Read the model definition and answer for the solid it produces. Units are mm, in the model's axes. Coordinates: 2 decimals unless noted, no trailing zeros. Write each loop counter-clockwise with the first axis right and the second up, starting at its lowest first coordinate (ties: lowest second). Pieces come first, ordered by that corner, then holes. Notation, with made-up numbers: (52, 19.5) -> (82, 19.5) arc R24 cw to (82, 54.5) -> close; hole circle Ø3 at (14, 65.5). An arc over 180 degrees is marked (long way). Return JSON: item names as keys, results as strings.
from build123d import *

# Parameters (mm, degrees)
F0_R      = 1.25
F1_DEPTH  = 6
F2_DEPTH  = 50
F3_DEPTH  = 50
F4_R      = 1.25
F5_DEPTH  = 6
F6_R      = 1.25
F7_DEPTH  = 6
F9_DEPTH  = 2
F11_DEPTH = 1.5
F10_W     = 6
F10_H     = 6
F12_DEPTH = 6
F13_R     = 1.25
F14_DEPTH = 30


with BuildPart() as f1:
    # F0 (on Top) → F1 (new body)
    with BuildSketch(Plane.XY):
        with BuildLine():
            ThreePointArc((10, -3), (12.1213203436, -2.1213203436), (13, 0))
            ThreePointArc((13, 0), (12.1213203436, 2.1213203436), (10, 3))
            ThreePointArc((10, 3), (7.8786796564, 2.1213203436), (7, 0))
            ThreePointArc((7, 0), (7.8786796564, -2.1213203436), (10, -3))
        make_face()
        with Locations((10, 0)):
            Circle(F0_R, mode=Mode.SUBTRACT)
        with BuildLine():
            ThreePointArc((7, 0), (7.8786796564, 2.1213203436), (10, 3))
            Line((10, 3), (7, 3))
            Line((7, 3), (7, 0))
        make_face()
        with BuildLine():
            Line((7, -3), (10, -3))
            ThreePointArc((10, -3), (7.8786796564, -2.1213203436), (7, 0))
            Line((7, 0), (7, -3))
        make_face()
        with BuildLine():
            Line((13, -3), (13, 0))
            ThreePointArc((13, 0), (12.1213203436, -2.1213203436), (10, -3))
            Line((10, -3), (13, -3))
        make_face()
        with BuildLine():
            ThreePointArc((10, 3), (12.1213203436, 2.1213203436), (13, 0))
            Line((13, 0), (13, 3))
            Line((13, 3), (10, 3))
        make_face()
        with Locations((10, 0)):
            Circle(F0_R)
    extrude(amount=F1_DEPTH)

    # F0 (on Top) → F2 (join)
    with BuildSketch(Plane.XY):
        with BuildLine():
            ThreePointArc((10, -3), (12.1213203436, -2.1213203436), (13, 0))
            ThreePointArc((13, 0), (12.1213203436, 2.1213203436), (10, 3))
            ThreePointArc((10, 3), (7.8786796564, 2.1213203436), (7, 0))
            ThreePointArc((7, 0), (7.8786796564, -2.1213203436), (10, -3))
        make_face()
        with Locations((10, 0)):
            Circle(F0_R, mode=Mode.SUBTRACT)
    extrude(amount=F2_DEPTH)

    # F4 (on face) → F5 (cut)
    with BuildSketch(Plane.YZ.offset(13)):
        with Locations((0, 3)):
            Circle(F4_R)
        with BuildLine():
            Line((-3, 0), (0, 0))
            ThreePointArc((0, 0), (-2.1213203436, 0.8786796564), (-3, 3))
            Line((-3, 3), (-3, 0))
        make_face()
        with BuildLine():
            Line((3, 0), (3, 3))
            ThreePointArc((3, 3), (2.1213203436, 0.8786796564), (0, 0))
            Line((0, 0), (3, 0))
        make_face()
    extrude(amount=-F5_DEPTH, mode=Mode.SUBTRACT)



with BuildPart() as f1b:
    # F0 (on Top) → F1, piece 2 (new body)
    with BuildSketch(Plane.XY):
        with BuildLine():
            ThreePointArc((-10, 3), (-7.8786796564, 2.1213203436), (-7, 0))
            Line((-7, 0), (-7, 3))
            Line((-7, 3), (-10, 3))
        make_face()
        with BuildLine():
            ThreePointArc((-13, 0), (-12.1213203436, 2.1213203436), (-10, 3))
            Line((-10, 3), (-13, 3))
            Line((-13, 3), (-13, 0))
        make_face()
        with BuildLine():
            ThreePointArc((-10, -3), (-7.8786796564, -2.1213203436), (-7, 0))
            ThreePointArc((-7, 0), (-7.8786796564, 2.1213203436), (-10, 3))
            ThreePointArc((-10, 3), (-12.1213203436, 2.1213203436), (-13, 0))
            ThreePointArc((-13, 0), (-12.1213203436, -2.1213203436), (-10, -3))
        make_face()
        with Locations((-10, 0)):
            Circle(F0_R, mode=Mode.SUBTRACT)
        with BuildLine():
            Line((-13, -3), (-10, -3))
            ThreePointArc((-10, -3), (-12.1213203436, -2.1213203436), (-13, 0))
            Line((-13, 0), (-13, -3))
        make_face()
        with BuildLine():
            Line((-7, -3), (-7, 0))
            ThreePointArc((-7, 0), (-7.8786796564, -2.1213203436), (-10, -3))
            Line((-10, -3), (-7, -3))
        make_face()
        with Locations((-10, 0)):
            Circle(F0_R)
    extrude(amount=F1_DEPTH)

    # F0 (on Top) → F3 (join)
    with BuildSketch(Plane.XY):
        with BuildLine():
            ThreePointArc((-10, -3), (-7.8786796564, -2.1213203436), (-7, 0))
            ThreePointArc((-7, 0), (-7.8786796564, 2.1213203436), (-10, 3))
            ThreePointArc((-10, 3), (-12.1213203436, 2.1213203436), (-13, 0))
            ThreePointArc((-13, 0), (-12.1213203436, -2.1213203436), (-10, -3))
        make_face()
        with Locations((-10, 0)):
            Circle(F0_R, mode=Mode.SUBTRACT)
    extrude(amount=F3_DEPTH)

    # F6 (on face) → F7 (cut)
    with BuildSketch(Plane(origin=(-13, 0, 0), x_dir=(0, -1, 0), z_dir=(-1, 0, 0))):
        with Locations((0, 3)):
            Circle(F6_R)
        with BuildLine():
            Line((-3, 0), (0, 0))
            ThreePointArc((0, 0), (-2.1213203436, 0.8786796564), (-3, 3))
            Line((-3, 3), (-3, 0))
        make_face()
        with BuildLine():
            Line((3, 0), (3, 3))
            ThreePointArc((3, 3), (2.1213203436, 0.8786796564), (0, 0))
            Line((0, 0), (3, 0))
        make_face()
    extrude(amount=-F7_DEPTH, mode=Mode.SUBTRACT)


with BuildPart() as f9:
    # F8 (on Front) → F9 (new body, symmetric)
    with BuildSketch(Plane.XZ):
        Polygon((-10, 7), (10, 7), (10, 11), (7.5421927808, 11), (-7.5421927808, 11), (-10, 11), align=None)
    extrude(amount=F9_DEPTH, both=True)


with BuildPart() as f1_1:
    add(f1.part)

    add(f1b.part)  # F11 merges F1b

    add(f9.part)  # F11 merges F9
    # F8 (on Front) → F11 (join, symmetric)
    with BuildSketch(Plane.XZ):
        Polygon((-10, 39), (-10, 35.5590698932), (-2.4578072192, 25), (0, 28.4409301068), (-7.5421927808, 39), align=None)
        Polygon((-2.4578072192, 25), (0, 21.5590698932), (2.4578072192, 25), (0, 28.4409301068), align=None)
        Polygon((7.5421927808, 11), (10, 11), (10, 14.4409301068), (2.4578072192, 25), (0, 21.5590698932), align=None)
        Polygon((-10, 14.4409301068), (-10, 11), (-7.5421927808, 11), (0, 21.5590698932), (-2.4578072192, 25), align=None)
        Polygon((2.4578072192, 25), (10, 35.5590698932), (10, 39), (7.5421927808, 39), (0, 28.4409301068), align=None)
        Polygon((7.5421927808, 39), (10, 39), (10, 43), (-10, 43), (-10, 39), (-7.5421927808, 39), align=None)
    extrude(amount=F11_DEPTH, both=True)

    # F10 (on face) → F12 (join)
    with BuildSketch(Plane.XY.offset(50)):
        with Locations((-10, 0)):
            Rectangle(F10_W, F10_H)
        with Locations((10, 0)):
            Rectangle(F10_W, F10_H)
    extrude(amount=-F12_DEPTH)

    # F13 (on face) → F14 (cut)
    with BuildSketch(Plane.YZ.offset(13)):
        with Locations((0, 47)):
            Circle(F13_R)
        with BuildLine():
            Line((-3, 50), (-3, 47))
            ThreePointArc((-3, 47), (-2.1213203436, 49.1213203436), (0, 50))
            Line((0, 50), (-3, 50))
        make_face()
        with BuildLine():
            ThreePointArc((0, 50), (2.1213203436, 49.1213203436), (3, 47))
            Line((3, 47), (3, 50))
            Line((3, 50), (0, 50))
        make_face()
    extrude(amount=-F14_DEPTH, mode=Mode.SUBTRACT)


solid = f1_1.part
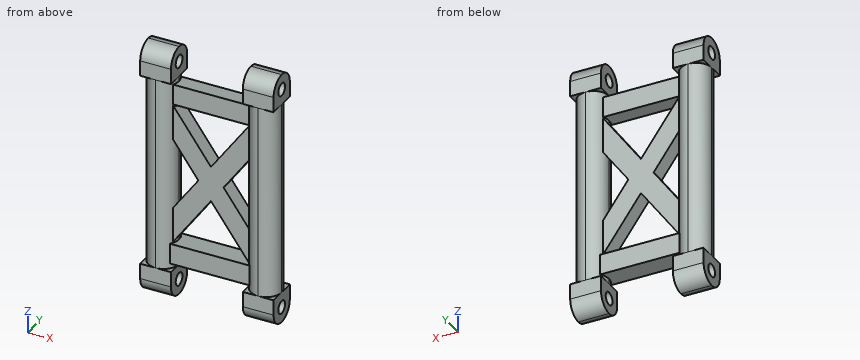
1. Consider L1, parallel to X at y = -0.25, z = 19; L2, parallel to Y at x = -10, z = 25.5; L3, parallel to X at y = -1, z = 19.5. Determine where each line is inside the solid, lowest interval first.
Taken from the geometry:
{"L1": "x = -12.99 to -11.22, -8.78 to -7.01, -6.74 to -1.83, 1.83 to 6.74, 7.01 to 8.78, 11.22 to 12.99", "L2": "y = -3 to -1.25, 1.25 to 3", "L3": "x = -12.83 to -10.75, -9.25 to -7.17, -6.39 to -1.47, 1.47 to 6.39, 7.17 to 9.25, 10.75 to 12.83"}
2. The part is cut by section D-D (z = 17.5). Determine the outline of the cut face in (x, y), then the cut area to 3 significant figures.
Taken from the geometry:
{"outline": "(-7.4, -1.5) -> (-2.9, -1.5) -> (-2.9, 1.5) -> (-7.4, 1.5) arc R3 ccw (long way) to start; (2.9, -1.5) -> (7.4, -1.5) arc R3 ccw (long way) to (7.4, 1.5) -> (2.9, 1.5) -> close; hole circle Ø2.5 at (-10, 0); hole circle Ø2.5 at (10, 0)", "area": "72.1 mm2"}
3. The part is cut by section C-C (z = 46.5). Determine the outline of the cut face in (x, y).
Taken from the geometry:
{"outline": "(-13, -3) -> (-7, -3) -> (-7, -1.15) -> (-13, -1.15) -> close; (-13, 1.15) -> (-7, 1.15) -> (-7, 3) -> (-13, 3) -> close; (7, -3) -> (13, -3) -> (13, -1.15) -> (7, -1.15) -> close; (7, 1.15) -> (13, 1.15) -> (13, 3) -> (7, 3) -> close"}
4. Flat-ended cylindrical pins translate along their axes: pin 1 Ø6 at (x, z) = (8, 26.5) entering from +Y; pin 2 Ø1.5 at (x, z) = (3.5, 34) entering from -Y; pin 3 Ø1.5 at (x, z) = (-2.5, 20) entering from +Y; pin 4 Ø2.5 at (x, y) = (-8.5, 1.5) entering from +Z. Find the tip coordinate at first contact, or state that the pin passes through.
Taken from the geometry:
{"pin 1": "stops at y = 3", "pin 2": "stops at y = -1.5", "pin 3": "stops at y = 1.5", "pin 4": "stops at z = 49.99"}
5. The part is cut by section A-A (z = 6.5). Determine the outline of the cut face in (x, y), then the cut area to 3 significant figures.
Taken from the geometry:
{"outline": "circle Ø6 at (-10, 0); circle Ø6 at (10, 0); hole circle Ø2.5 at (-10, 0); hole circle Ø2.5 at (10, 0)", "area": "46.7 mm2"}
6. The part is cut by section B-B (z = 30.5). Determine the outline of the cut face in (x, y).
Taken from the geometry:
{"outline": "circle Ø6 at (-10, 0); (-6.39, -1.5) -> (-1.47, -1.5) -> (-1.47, 1.5) -> (-6.39, 1.5) -> close; (1.47, -1.5) -> (6.39, -1.5) -> (6.39, 1.5) -> (1.47, 1.5) -> close; circle Ø6 at (10, 0); hole circle Ø2.5 at (-10, 0); hole circle Ø2.5 at (10, 0)"}
